from build123d import *

# Parameters (mm, degrees)
SKETCH2_R           = 9.5
SKETCH2_R_2         = 5.15
BOSS_EXTRUDE1_DEPTH = 3
BOSS_EXTRUDE2_DEPTH = 2
SKETCH4_R           = 5.15
BOSS_EXTRUDE3_DEPTH = 3
SKETCH5_R           = 0.5
CUT_EXTRUDE1_DEPTH  = 14.765899898
SKETCH6_R           = 9.5
CUT_EXTRUDE2_DEPTH  = 0.65


with BuildPart() as part:
    # Sketch2 → Boss-Extrude1 (new body)
    with BuildSketch(Plane.XY):
        Circle(SKETCH2_R)
        Circle(SKETCH2_R_2, mode=Mode.SUBTRACT)
    extrude(amount=BOSS_EXTRUDE1_DEPTH)

    # Sketch3 → Boss-Extrude2 (add)
    with BuildSketch(Plane.XY.offset(3)):
        with BuildLine():
            Line((6.143973875, -5.278407433), (6.275470836, -5.125347271))
            Line((6.275470836, -5.125347271), (4.527710902, -2.882271968))
            Line((4.527710902, -2.882271968), (1.687974032, -5.0949388))
            Line((1.687974032, -5.0949388), (3.435733966, -7.338014103))
            Line((3.435733966, -7.338014103), (3.616296002, -7.247924063))
            ThreePointArc((3.616296002, -7.247924063), (4.978500372, -6.389407957), (6.143973875, -5.278407433))
        make_face()
        with BuildLine():
            Line((-8.085034364, 0.691867379), (-5.256333448, 1.085641007))
            Line((-5.256333448, 1.085641007), (-4.759976196, -2.479976678))
            Line((-4.759976196, -2.479976678), (-7.576416358, -2.872043529))
            Line((-7.576416358, -2.872043529), (-7.643221866, -2.68163374))
            ThreePointArc((-7.643221866, -2.68163374), (-8.022639792, -1.116803816), (-8.085034364, 0.492157827))
            Line((-8.085034364, 0.492157827), (-8.085034364, 0.691867379))
        make_face()
        with BuildLine():
            Line((3.742806644, 3.938550831), (4.68847999, 6.609921942))
            Line((4.68847999, 6.609921942), (4.479502253, 6.748633904))
            ThreePointArc((4.479502253, 6.748633904), (3.050121393, 7.503783012), (1.499247991, 7.960041172))
            Line((1.499247991, 7.960041172), (1.300945522, 7.9973908))
            Line((1.300945522, 7.9973908), (0.232265294, 5.362248647))
            Line((0.232265294, 5.362248647), (3.742806644, 3.938550831))
        make_face()
    extrude(amount=BOSS_EXTRUDE2_DEPTH)

    # Sketch4 → Boss-Extrude3 (add)
    with BuildSketch(Plane(origin=(0, 0, 0), x_dir=(-1, 0, 0), z_dir=(0, 0, -1))):
        Circle(SKETCH4_R)
    extrude(amount=-BOSS_EXTRUDE3_DEPTH)

    # Sketch5 → Cut-Extrude1 (cut, through all)
    with BuildSketch(Plane.XY.offset(3)):
        with Locations((2.745365917, -3.523402937)):
            Circle(SKETCH5_R)
        with Locations((1.79878696, -4.260958548)):
            Circle(SKETCH5_R)
        with Locations(Location((3.691944873, -2.785847327, 0), (0, 0, 180))):
            Circle(SKETCH5_R)
        with Locations(Location((0.566642119, 4.590241713, 0), (0, 0, 180))):
            Circle(SKETCH5_R)
        with Locations(Location((1.678673493, 4.139258095, 0), (0, 0, 180))):
            Circle(SKETCH5_R)
        with Locations((2.790704867, 3.688274478)):
            Circle(SKETCH5_R)
        with Locations(Location((-4.258586993, -1.804394387, 0), (0, 0, 180))):
            Circle(SKETCH5_R)
        with Locations(Location((-4.42403941, -0.615855158, 0), (0, 0, 180))):
            Circle(SKETCH5_R)
        with Locations((-4.589491827, 0.57268407)):
            Circle(SKETCH5_R)
    extrude(amount=-CUT_EXTRUDE1_DEPTH, mode=Mode.SUBTRACT)

    # Sketch6 → Cut-Extrude2 (cut)
    with BuildSketch(Plane(origin=(0, 0, 0), x_dir=(-1, 0, 0), z_dir=(0, 0, -1))):
        Circle(SKETCH6_R)
    extrude(amount=-CUT_EXTRUDE2_DEPTH, mode=Mode.SUBTRACT)


solid = part.part
Could you check a few things on this model? Use its own coordinates, in mm. A direction names the side the tool comes from. Give positions to 0.01 mm unless a question says otherwise; leave off trailing zeros. Write each loop counter-clockwise with the first axis right and the second up, starting at its lowest first coordinate (ties: lowest second). Pieces come first, ordered by that corner, then holes. Notation, with made-up numbers: (53.5, -22.5) -> (103.5, -22.5) arc R12 ccw to (103.5, -8.5) -> close; hole circle Ø2 at (56.5, 4.5). An arc over 180 degrees is marked (long way). Write each question's results on one line, items separated by ' | '. Start each with the question number.
Q1. I'm going to push flat-ended pins straight in: pin 1 Ø8 at (x, y) = (5.5, 4.5) entering from +Z; pin 2 Ø1 at (y, z) = (6, 1.5) entering from -X. Where does each tip first touch, or does it pass through?
Q2. Which directions (+Z, -Z, +X, -X, +Y, -Y) give clear straight access to the entire face, cutting with the end or side of a thin tool? Please do faces 5 (the face through (3.13, -3.97, 3.99)), 6 (the face through (4.961, -6.403, 3.986)), 7 (the face through (3.071, 7.495, 3.986)), 8 (the face through (2.55, -6.2, 3.99)).
Q3. I need wall thicknesses on probe 1 along Y at (x, z) = (3, 1); probe 2 along Z at (x, y) = (-2.5, 7.75); probe 3 along X at (y, z) = (3.75, 0.95). Which ranges of each line are inside material? Lowest first, please.
Q4. We'd pull the mould along Y, two halves only. Please class faces 1 (the face through (4.38, -8.43, 1.81)), 2 (the face through (-4.03, -0.31, 1.84)), 3 (the face through (2, 6, 5)), 4 (the face through (-6.148, -2.673, 3.986)): +Y half, -Y half, draft (parallel to the pull), parting line (faces both ways), or undercut.
Q5. Suppose I cut it at B-B, the plane z = 2.45. State how many separate pieces and enclosed holes the cut face has, and give its area (3 significant figures).
Q6. Suppose I cut it at A-A, the plane x = -5.75. List the corners of the cut face in (y, z) for me, and give its area (3 significant figures).
Outcome:
1) pin 1: z = 5 | pin 2: x = -7.75
2) face 5: +Z, -X | face 6: +Z, +X, -Y | face 7: +Z, +X, +Y | face 8: +Z, -X, -Y
3) probe 1: -9.01 to -3.95, -3.09 to 3.23, 4.14 to 9.01 | probe 2: 0.65 to 3 | probe 3: -8.73 to 1.36, 1.99 to 2.29, 3.29 to 8.73
4) face 1: parting line | face 2: undercut | face 3: draft | face 4: -Y half
5) separate pieces: 1 | enclosed holes: 9 | area: 276 mm2
6) outline: (-7.56, 0.65) -> (7.56, 0.65) -> (7.56, 3) -> (1.02, 3) -> (1.02, 5) -> (-2.62, 5) -> (-2.62, 3) -> (-7.56, 3) -> close | area: 42.8 mm2
